Source: CAD feature listing. Evaluate the final solid. Frame: model axes, mm. Round coordinates to 2 decimals unless told otherwise and drop trailing zeros. Order: outer loops, then holes, each group sorted by start corner. A loop starts at its lowest first (then second) coordinate and runs counter-clockwise, first axis right, second up. Notation, with made-up numbers: M 4,-26.75 L 12,-26.75 A20 ccw 12,1.25 Z; hole C 34.25,62 d11. An arc over 180 degrees is marked long. Answer in a Markdown table with one row per item. Add a question column.
```python
from build123d import *

# Parameters (mm, degrees)
F0_W     = 35.12583673
F0_H     = 34.2667922378
F1_DEPTH = 25
F2_R     = 5
F3_D     = 10.3


with BuildPart() as f1:
    # F0 (on Front) → F1 (new body)
    with BuildSketch(Plane.XZ):
        Rectangle(F0_W, F0_H)
    extrude(amount=F1_DEPTH)

    # F2
    f2_edges = [f1.edges().sort_by_distance(p)[0] for p in [
        (17.562918, -12.5, 17.133396),
    ]]
    fillet(f2_edges, radius=F2_R)

    # F3 (through all)
    with Locations(Plane(origin=(0, 0, 0), x_dir=(1, 0, 0), z_dir=(0, 1, 0))):
        with Locations((0, 0)):
            Hole(F3_D / 2)


solid = f1.part
```
(1) Cut plane A-A (x = 0). Return loops of the section in (y, z), and give its area (3 significant figures).
(2) Line query: line 1 (Z direction, x = 0, y = -6.25); line 2 (X direction, y = -18.75, z = 1); line 3 (Z direction, x = 4, y = -23.25). Output: solid intervals per line, ascending. Write a range as from..to.
(3) Cut plane B-B (z = 0). Return loops of the section in (x, y), and give its area (3 significant figures).
(4) Cut plane C-C (y = -9.5). Return loops of the section in (x, z).
(5) Pin query (flat end, axial travel): pin 1 (12 mm diameter, centred on x = 0, z = 0, fed in from -Y). Return the tip coordinate at first contact, or that it passes through.
(6) Draft query along Z for faces 1 (the face through (-4.91, -12.68, -1.55)), 2 (the face through (0, -12, -17.133)), 3 (the face through (16.137, -12.675, 15.63)), 4 (the face through (17.563, -12, -3)). Return one class per face: +Z half, -Z half, draft (parallel to the pull), parting line (faces both ways), or undercut.
Answer list:
| question | item | result |
|---|---|---|
| 1 | outline | M -25,-17.13 L 0,-17.13 L 0,-5.15 L -25,-5.15 Z; M -25,5.15 L 0,5.15 L 0,17.13 L -25,17.13 Z |
| 1 | area | 599 mm² |
| 2 | line 1 | -17.13..-5.15, 5.15..17.13 |
| 2 | line 2 | -17.56..-5.05, 5.05..17.56 |
| 2 | line 3 | -17.13..-3.24, 3.24..17.13 |
| 3 | outline | M -17.56,-25 L -5.15,-25 L -5.15,0 L -17.56,0 Z; M 5.15,-25 L 17.56,-25 L 17.56,0 L 5.15,0 Z |
| 3 | area | 621 mm² |
| 4 | outline | M -17.56,-17.13 L 17.56,-17.13 L 17.56,12.13 A5 ccw 12.56,17.13 L -17.56,17.13 Z; hole C 0,0 d10.3 |
| 5 | pin 1 | y = -25 |
| 6 | face 1 | undercut |
| 6 | face 2 | -Z half |
| 6 | face 3 | +Z half |
| 6 | face 4 | draft |
